Can you work these out from the model? Positions are in its coordinate system, mm. Face numbers are marked on the shaded views. A direction names the side the tool comes from. Round coordinates to 2 decimals unless told otherwise and drop trailing zeros. Loops run counter-clockwise (first coordinate to the right, second up) from the corner with the lowest first, then second, coordinate; pieces in that order, holes last.
(1) Which directions (+Z, -Z, +X, -X, +Y, -Y) give clear straight access to the entire face, cutting with the end or side of a thin tool? Please do the marked faces 1 and 2.
(2) Thinking about a two-plate mould opening in Y: for the marked faces 3, 4 and 5, which applies, released by +Y, released by -Y, zero draft, split by the parting line, or undercut?
(3) I want a section at A-A on x = 0. Write out the boundary of the cut face in (y, z), plus the area to 3 significant figures.
(4) I want a section at D-D on x = -7.5. Write out the boundary of the cut face in (y, z).
(5) Will these pins go through, and if not, where does the flat tip stop? pin 1 Ø2 at (x, z) = (13.5, 11) entering from -Y; pin 2 Ø4 at (x, y) = (0.5, -3) entering from +Z; pin 3 Ø12 at (x, z) = (3, 35.5) entering from -Y.
(6) If I drill on line 1 along Y through (x, z) = (0, 37.75); line 2 along Z through (x, y) = (10.5, 7.5); line 3 along Z through (x, y) = (4, 3.5), over which ranges is the centre line in solid material (lowest first)?
(7) I want a section at C-C on z = 7.5. Write out the boundary of the cut face in (x, y).
from build123d import *

# Parameters (mm, degrees)
F0_R     = 10
F0_R_2   = 6.75
F1_DEPTH = 42
F0_R_3   = 12
F2_DEPTH = 32
F0_R_4   = 18
F3_DEPTH = 20


with BuildPart() as f1:
    # F0 (on Top) → F1 (new body)
    with BuildSketch(Plane.XY):
        Circle(F0_R)
        Circle(F0_R_2, mode=Mode.SUBTRACT)
    extrude(amount=F1_DEPTH)

    # F0 (on Top) → F2 (join)
    with BuildSketch(Plane.XY):
        Circle(F0_R_3)
        Circle(F0_R, mode=Mode.SUBTRACT)
        Circle(F0_R_2)
    extrude(amount=F2_DEPTH)

    # F0 (on Top) → F3 (join)
    with BuildSketch(Plane.XY):
        Circle(F0_R_4)
        Circle(F0_R_3, mode=Mode.SUBTRACT)
    extrude(amount=F3_DEPTH)


solid = f1.part
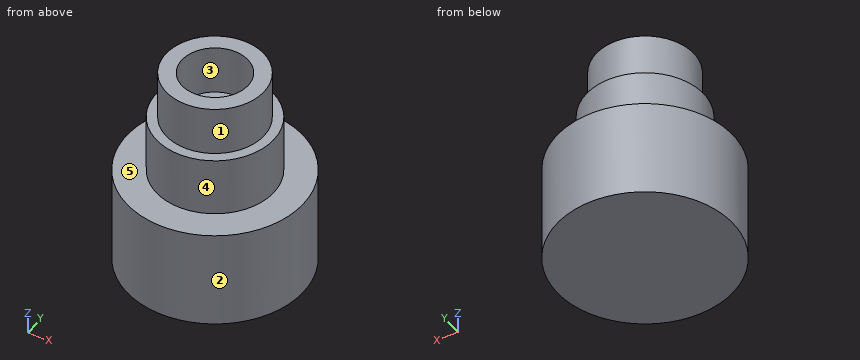
Filled sheet:
1. face 1: +Z
1. face 2: +Z, -Z
2. face 3: undercut
2. face 4: split by the parting line
2. face 5: zero draft
3. outline: (-18, 0) - (18, 0) - (18, 20) - (12, 20) - (12, 32) - (10, 32) - (10, 42) - (6.75, 42) - (6.75, 32) - (-6.75, 32) - (-6.75, 42) - (-10, 42) - (-10, 32) - (-12, 32) - (-12, 20) - (-18, 20) - close
3. area: 1,070 mm2
4. outline: (-16.36, 0) - (16.36, 0) - (16.36, 20) - (9.37, 20) - (9.37, 32) - (6.61, 32) - (6.61, 42) - (-6.61, 42) - (-6.61, 32) - (-9.37, 32) - (-9.37, 20) - (-16.36, 20) - close
5. pin 1: stops at y = -12.95
5. pin 2: stops at z = 32
5. pin 3: stops at y = -12
6. line 1: y = -10 to -6.75, 6.75 to 10
6. line 2: z = 0 to 20
6. line 3: z = 0 to 32
7. outline: circle Ø36 at (0, 0)
